from build123d import *

# Parameters (mm, degrees)
F0_W      = 12.4007742852
F0_H      = 147.8563919663
F1_DEPTH  = 12.7
F2_W      = 12.4007742852
F2_H      = 7.5796097517
F2_H_2    = 7.3651988059
F2_H_3    = 7.48882466
F2_H_4    = 7.4724052101
F2_H_5    = 7.208738476
F2_H_6    = 7.6124407351
F2_H_7    = 7.3697865009
F3_DEPTH  = 17.78
F4_W      = 12.4007742852
F4_H      = 4.9358203965
F5_DEPTH  = 6.35
F6_W      = 12.4007742852
F6_H      = 5.8721274096
F8_W      = 12.4007742852
F8_H      = 4.2509499896
F9_W      = 12.4007742852
F9_H      = 4.4994622427
F10_W     = 12.4007742852
F10_H     = 4.5405410188
F11_W     = 12.4007742852
F11_H     = 5.0489034462
F12_DEPTH = 6.35
F7_W      = 12.4007742852
F7_H      = 4.9657884943
F13_DEPTH = 6.35


with BuildPart() as f1:
    # F0 (on Top) → F1 (new body)
    with BuildSketch(Plane.XY):
        with Locations((-36.0559495166, 0.0271089375)):
            Rectangle(F0_W, F0_H)
    extrude(amount=F1_DEPTH)

    # F2 (on face) → F3 (join)
    with BuildSketch(Plane.XY.offset(12.7)):
        with Locations((-36.0559495166, -47.0269694924)):
            Rectangle(F2_W, F2_H)
        with Locations((-36.0559495166, -23.3870735392)):
            Rectangle(F2_W, F2_H_2)
        with Locations((-36.0559495166, -1.4402301749)):
            Rectangle(F2_W, F2_H_3)
        with Locations((-36.0559495166, 19.5383997634)):
            Rectangle(F2_W, F2_H_4)
        with Locations((-36.0559495166, 42.6099169999)):
            Rectangle(F2_W, F2_H_5)
        with Locations((-36.0559495166, 64.5896028727)):
            Rectangle(F2_W, F2_H_6)
        with Locations((-36.0559495166, -70.2161937952)):
            Rectangle(F2_W, F2_H_7)
    extrude(amount=F3_DEPTH)

    # F4 (on face) → F5 (join)
    with BuildSketch(Plane(origin=(0, -66.5313005447, 0), x_dir=(-1, 0, 0), z_dir=(0, 1, 0))):
        with Locations((36.0559495166, 28.0120898017)):
            Rectangle(F4_W, F4_H)
    extrude(amount=F5_DEPTH)

    # F6 (on face) + F8 (on face) + F9 (on face) + F10 (on face) + F11 (on face) → F12 (join)
    with BuildSketch(Plane(origin=(0, -43.2371646166, 0), x_dir=(-1, 0, 0), z_dir=(0, 1, 0))):
        with Locations((36.0559495166, 27.5439362952)):
            Rectangle(F6_W, F6_H)
    with BuildSketch(Plane(origin=(0, 2.3041821551, 0), x_dir=(-1, 0, 0), z_dir=(0, 1, 0))):
        with Locations((36.0559495166, 28.3545250052)):
            Rectangle(F8_W, F8_H)
    with BuildSketch(Plane(origin=(0, 23.2746023685, 0), x_dir=(-1, 0, 0), z_dir=(0, 1, 0))):
        with Locations((36.0559495166, 28.2302688786)):
            Rectangle(F9_W, F9_H)
    with BuildSketch(Plane(origin=(0, 46.214286238, 0), x_dir=(-1, 0, 0), z_dir=(0, 1, 0))):
        with Locations((36.0559495166, 28.2097294906)):
            Rectangle(F10_W, F10_H)
    with BuildSketch(Plane(origin=(0, 68.3958232403, 0), x_dir=(-1, 0, 0), z_dir=(0, 1, 0))):
        with Locations((36.0559495166, 27.9555482769)):
            Rectangle(F11_W, F11_H)
    extrude(amount=F12_DEPTH)

    # F7 (on face) → F13 (join)
    with BuildSketch(Plane(origin=(0, -19.7044741362, 0), x_dir=(-1, 0, 0), z_dir=(0, 1, 0))):
        with Locations((36.0559495166, 27.9971057528)):
            Rectangle(F7_W, F7_H)
    extrude(amount=F13_DEPTH)


solid = f1.part
Part model, mm, in its own coordinate system. A direction names the side the tool comes from. Coordinates: 2 decimals unless noted, no trailing zeros. Order: outer loops, then holes, each group sorted by start corner. A loop starts at its lowest first (then second) coordinate and runs counter-clockwise, first axis right, second up. Notation, with made-up numbers: M 40,63 L 47,63 A5 ccw 47,67 Z; hole C -35.5,-15.5 d8. An arc over 180 degrees is marked long. Use a Markdown table: item, result.
(1) Tool access for faces 1 (the flat face through (-36, 2, 30.48)), 2 (the flat face through (-36, 39.006, 21)), 3 (the flat face through (-36, 23.275, 19)), 4 (the flat face through (-36, 68.396, 19)): list every direction of +Z, -Z, +X, -X, +Y, -Y with a clear straight run to the whole face (end or side of a thin tool).
A:
| item | result |
|---|---|
| face 1 | +Z, +X, -X, +Y, -Y |
| face 2 | +Z, +X, -X |
| face 3 | +X, -X |
| face 4 | +X, -X, +Y |
(2) Probe L1, parallel to Z at x = -36, y = -16; L2, parallel to Z at x = -31.5, y = 49; L3, parallel to Y at x = -35.5, z = 8. List the from-to ranges inside material, lowest first.
A:
| item | result |
|---|---|
| L1 | z = 0 to 12.7, 25.51 to 30.48 |
| L2 | z = 0 to 12.7, 25.94 to 30.48 |
| L3 | y = -73.9 to 73.96 |
(3) Cut at A-A on z = 16. Write the cut outline in (x, y), then the cut area to 3 significant figures.
A:
| item | result |
|---|---|
| outline | M -42.26,-73.9 L -29.86,-73.9 L -29.86,-66.53 L -42.26,-66.53 Z; M -42.26,-50.82 L -29.86,-50.82 L -29.86,-43.24 L -42.26,-43.24 Z; M -42.26,-27.07 L -29.86,-27.07 L -29.86,-19.7 L -42.26,-19.7 Z; M -42.26,-5.18 L -29.86,-5.18 L -29.86,2.3 L -42.26,2.3 Z; M -42.26,15.8 L -29.86,15.8 L -29.86,23.27 L -42.26,23.27 Z; M -42.26,39.01 L -29.86,39.01 L -29.86,46.21 L -42.26,46.21 Z; M -42.26,60.78 L -29.86,60.78 L -29.86,68.4 L -42.26,68.4 Z |
| area | 646 mm^2 |
(4) Flat gauge pins, fed straight in: pin 1 (4 mm diameter, centred on x = -40, z = 4.5, fed in from +Y); pin 2 (3.5 mm diameter, centred on x = -34.5, z = 16.5, fed in from +Y). Where does each tip first touch, or does it go through?
A:
| item | result |
|---|---|
| pin 1 | stops at y = 73.96 |
| pin 2 | stops at y = 68.4 |
(5) Cut at C-C on y = 35.5. Write the cut outline in (x, z), then the cut area to 3 significant figures.
A:
| item | result |
|---|---|
| outline | M -42.26,0 L -29.86,0 L -29.86,12.7 L -42.26,12.7 Z |
| area | 157 mm^2 |
(6) Cut at B-B on y = -65. Write the cut outline in (x, z), then the cut area to 3 significant figures.
A:
| item | result |
|---|---|
| outline | M -42.26,0 L -29.86,0 L -29.86,12.7 L -42.26,12.7 Z; M -42.26,25.54 L -29.86,25.54 L -29.86,30.48 L -42.26,30.48 Z |
| area | 219 mm^2 |
(7) Pull direction Y, two halves, no side cores. Call faces 5 (the flat face through (-36, 74.746, 28)), 6 (the flat face through (-36, -73.901, 15)), 7 (the flat face through (-36, 72, 25.431)), 8 (the flat face through (-36, -40, 24.608)): released by +Y, released by -Y, zero draft, split by the parting line, or undercut.
A:
| item | result |
|---|---|
| face 5 | released by +Y |
| face 6 | released by -Y |
| face 7 | zero draft |
| face 8 | undercut |
